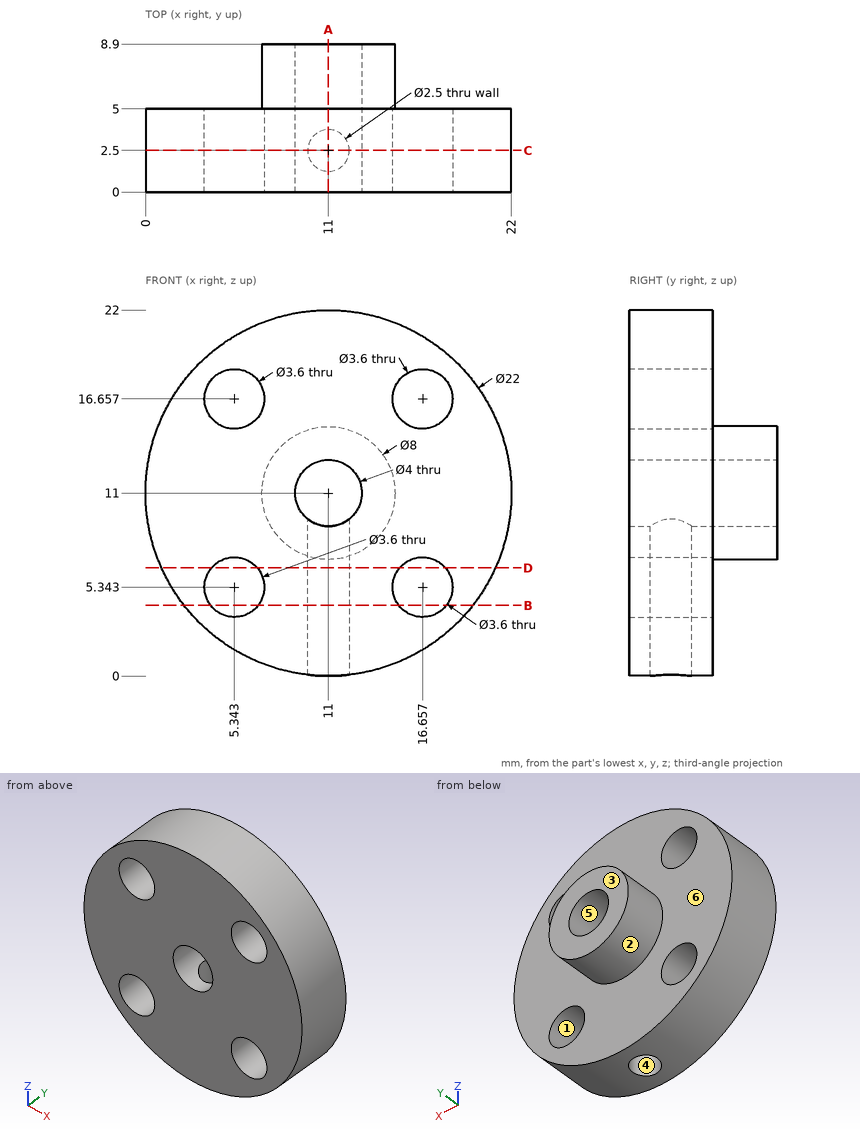
Geometry check sheet. Reference: drawing and pictorial views, mm from the part's lowest x, y, z. A direction names the side the tool comes from. Coordinates: 2 decimals unless noted, no trailing zeros. Order: outer loops, then holes, each group sorted by start corner. A loop starts at its lowest first (then second) coordinate and runs counter-clockwise, first axis right, second up.
Item 1: Section check A-A, the plane x = 11. Enter the section's corners in (y, z).
Filled in:
outline: (0, 0) - (1.25, 0) - (1.25, 9) - (0, 9) - close; (0, 13) - (8.9, 13) - (8.9, 15) - (5, 15) - (5, 22) - (0, 22) - close; (3.75, 0) - (5, 0) - (5, 7) - (8.9, 7) - (8.9, 9) - (3.75, 9) - close
Item 2: Section check D-D, the plane z = 6.5. Enter the section's corners in (x, y).
Filled in:
outline: (0.96, 0) - (3.96, 0) - (3.96, 5) - (0.96, 5) - close; (6.72, 0) - (15.28, 0) - (15.28, 5) - (6.72, 5) - close; (18.04, 0) - (21.04, 0) - (21.04, 5) - (18.04, 5) - close; hole circle Ø2.5 at (11, 2.5)
Item 3: Material ranges on L1, parallel to X at y = 2, z = 15.75; L2, parallel to Z at x = 11, y = 7.25; L3, parallel to Y at x = 11, z = 5.5, recorded low to high.
Filled in:
L1: x = 1.08 to 3.79, 6.9 to 15.1, 18.21 to 20.92
L2: z = 7 to 9, 13 to 15
L3: y = 0 to 1.25, 3.75 to 5
Item 4: Section check C-C, the plane y = 2.5. Enter the section's corners in (x, z), then the cut area to 3 significant figures.
Filled in:
outline: (9.75, 0.07) - (9.75, 9.44) arc R2 cw (long way) to (12.25, 9.44) - (12.25, 0.07) arc R11 ccw (long way) to start; hole circle Ø3.6 at (5.34, 5.34); hole circle Ø3.6 at (5.34, 16.66); hole circle Ø3.6 at (16.66, 5.34); hole circle Ø3.6 at (16.66, 16.66)
area: 304 mm2
Item 5: Depth check by flat-ended pin: pin 1 (4.5 mm diameter, centred on x = 16.66, z = 16.66, fed in from +Y); pin 2 (3 mm diameter, centred on x = 14, y = 6, fed in from -Z). Enter the tip coordinate at first touch or a pass-through.
Filled in:
pin 1: stops at y = 5
pin 2: stops at z = 0.16
Item 6: Section check B-B, the plane z = 4.25. Enter the section's corners in (x, y).
Filled in:
outline: (2.31, 0) - (3.91, 0) - (3.91, 5) - (2.31, 5) - close; (6.77, 0) - (15.23, 0) - (15.23, 5) - (6.77, 5) - close; (18.09, 0) - (19.69, 0) - (19.69, 5) - (18.09, 5) - close; hole circle Ø2.5 at (11, 2.5)
Item 7: Release check for a two-part mould opening along Z. For the marked faces 1, 2 and 3 record: +Z half, -Z half, draft (parallel to the pull), parting line (faces both ways), or undercut.
Filled in:
face 1: undercut
face 2: parting line
face 3: draft
Item 8: Access from +Z, -Z, +X, -X, +Y, -Y to the whole of each face (thin tool, end or side, straight path). Record for the marked faces 4, 5 and 6.
Filled in:
face 4: -Z
face 5: +Y, -Y
face 6: +Y
